Can you work these out from the drawing? Everything is in mm from the part's minimum corner. Round coordinates to 2 decimals unless told otherwise and drop trailing zeros. Write each loop counter-clockwise with the first axis right and the second up, starting at its lowest first coordinate (ties: lowest second). Pieces come first, ordered by that corner, then holes. Notation, with made-up numbers: (6, 7.5) - (24, 7.5) arc R17 ccw to (24, 39.5) - close; hole circle Ø11 at (73, -25.5). An arc over 180 degrees is marked (long way). One line per item, written item: value. Start each with the question number.
(1) If I drill on L1, parallel to X at y = 6.6, z = 43; L2, parallel to Y at x = 62.5, z = 80; L3, parallel to X at y = 5.05, z = 43, over which ranges is the centre line in solid material (lowest first)? Write a range as from..to.
(2) I want a section at B-B on y = 2. List the corners of the cut face in (x, z) for me.
(3) I want a section at D-D on x = 11. List the corners of the cut face in (y, z) for me.
(4) I want a section at A-A on x = 43. List the corners of the cut face in (y, z) for me, plus the area to 3 significant figures.
(5) I'm going to push flat-ended pins straight in: pin 1 Ø0.8 at (y, z) = (4, 37.5) entering from -X; pin 2 Ø3.5 at (x, y) = (43, 3) entering from +Z; pin 3 Ø4 at (x, y) = (67.5, 2) entering from +Z. Where does each tip first touch, or does it pass through?
(6) I want a section at C-C on z = 17.5. List the corners of the cut face in (x, y) for me.
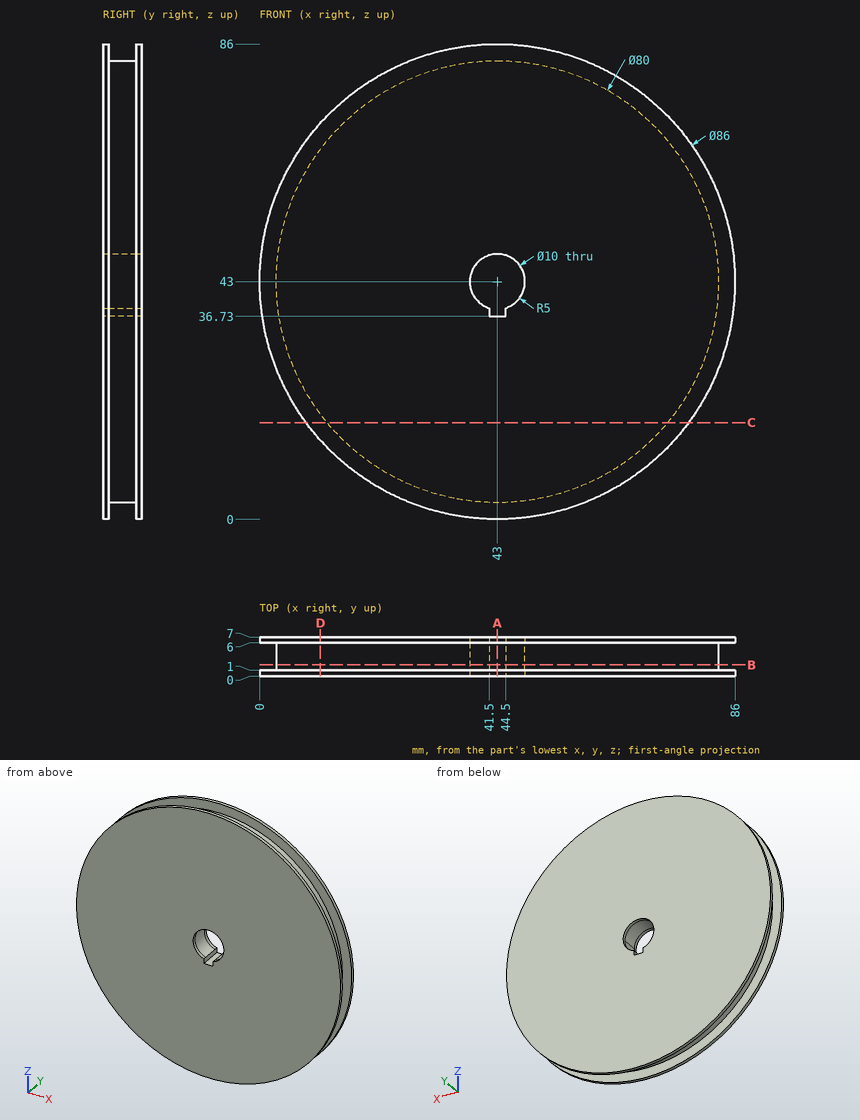
Established:
1. L1: 0..38, 48..86
1. L2: 0..1, 6..7
1. L3: 3..38, 48..83
2. outline: circle Ø80 at (43, 43); hole (41.5, 36.73) - (44.5, 36.73) - (44.5, 38.23) arc R5 ccw (long way) to (41.5, 38.23) - close
3. outline: (0, 14.28) - (1, 14.28) - (1, 19) - (6, 19) - (6, 14.28) - (7, 14.28) - (7, 71.72) - (6, 71.72) - (6, 67) - (1, 67) - (1, 71.72) - (0, 71.72) - close
4. outline: (0, 0) - (1, 0) - (1, 3) - (6, 3) - (6, 0) - (7, 0) - (7, 36.73) - (0, 36.73) - close; (0, 48) - (7, 48) - (7, 86) - (6, 86) - (6, 83) - (1, 83) - (1, 86) - (0, 86) - close
4. area: 493 mm2
5. pin 1: x = 3.33
5. pin 2: z = 83
5. pin 3: z = 79.48
6. outline: (8.38, 0) - (77.62, 0) - (77.62, 1) - (73.82, 1) - (73.82, 6) - (77.62, 6) - (77.62, 7) - (8.38, 7) - (8.38, 6) - (12.18, 6) - (12.18, 1) - (8.38, 1) - close
